from build123d import *

# Parameters (mm, degrees)
SKETCH1_W           = 14
SKETCH1_H           = 14
SKETCH1_W_2         = 9
SKETCH1_H_2         = 9
BOSS_EXTRUDE1_DEPTH = 2.5
SKETCH3_R           = 2.5
BOSS_EXTRUDE2_DEPTH = 3.4
SKETCH4_R           = 0.7
CUT_EXTRUDE1_DEPTH  = 5
FILLET1_R           = 1


with BuildPart() as part:
    # Sketch1 → Boss-Extrude1 (new body, symmetric)
    with BuildSketch(Plane.XY):
        Rectangle(SKETCH1_W, SKETCH1_H)
        Rectangle(SKETCH1_W_2, SKETCH1_H_2, mode=Mode.SUBTRACT)
    extrude(amount=BOSS_EXTRUDE1_DEPTH, both=True)

    # Sketch3 → Boss-Extrude2 (add)
    with BuildSketch(Plane(origin=(7, 0, 0), x_dir=(0, 0, -1), z_dir=(1, 0, 0))):
        Circle(SKETCH3_R)
    boss_extrude2 = extrude(amount=BOSS_EXTRUDE2_DEPTH)

    # Sketch4 → Cut-Extrude1 (cut)
    with BuildSketch(Plane(origin=(10.4, 0, 0), x_dir=(0, 0, -1), z_dir=(1, 0, 0))):
        Circle(SKETCH4_R)
    cut_extrude1 = extrude(amount=-CUT_EXTRUDE1_DEPTH, mode=Mode.SUBTRACT)

    # Mirror1: Boss-Extrude2, Cut-Extrude1 across plane
    add(boss_extrude2.mirror(Plane(origin=(0, 0, 0), x_dir=(0, 0, 1), z_dir=(1, 0, 0))))
    add(cut_extrude1.mirror(Plane(origin=(0, 0, 0), x_dir=(0, 0, 1), z_dir=(1, 0, 0))), mode=Mode.SUBTRACT)

    # Fillet1
    fillet1_edges = [part.edges().sort_by_distance(p)[0] for p in [
        (-7, 7, 0),
        (7, 7, 0),
        (7, -7, 0),
        (-7, -7, 0),
    ]]
    fillet(fillet1_edges, radius=FILLET1_R)


solid = part.part
Input: part model. Units: mm. Frame: model coordinates. A direction names the side the tool comes from. Round coordinates to 2 decimals unless told otherwise and drop trailing zeros. Order: outer loops, then holes, each group sorted by start corner. A loop starts at its lowest first (then second) coordinate and runs counter-clockwise, first axis right, second up.
1. Material intervals for line 1 (Y direction, x = 8.45, z = 0); line 2 (X direction, y = -1.5, z = -1.3); line 3 (X direction, y = -2, z = -1.9), sorted ascending.
The answers:
line 1: y = -2.5 to -0.7, 0.7 to 2.5
line 2: x = -10.4 to -4.5, 4.5 to 10.4
line 3: x = -7 to -4.5, 4.5 to 7
2. Set-up query: faces 4 (the face through (-5.4, 0, 0)), 5 (the face through (7.9, 0, 0.7)), 6 (the face through (4.5, 0, 0)). Return all of +Z, -Z, +X, -X, +Y, -Y with unobstructed straight access to the full face (end or side cutting, diameter ignored); none if empty.
The answers:
face 4: -X
face 5: +X
face 6: +Z, -Z
3. Cut plane B-B, the plane z = 0. Output: boundary loops of the cut face in (x, y).
The answers:
outline: (-10.4, -2.5) - (-7, -2.5) - (-7, -6) arc R1 ccw to (-6, -7) - (6, -7) arc R1 ccw to (7, -6) - (7, -2.5) - (10.4, -2.5) - (10.4, -0.7) - (5.4, -0.7) - (5.4, 0.7) - (10.4, 0.7) - (10.4, 2.5) - (7, 2.5) - (7, 6) arc R1 ccw to (6, 7) - (-6, 7) arc R1 ccw to (-7, 6) - (-7, 2.5) - (-10.4, 2.5) - (-10.4, 0.7) - (-5.4, 0.7) - (-5.4, -0.7) - (-10.4, -0.7) - close; hole (-4.5, -4.5) - (4.5, -4.5) - (4.5, 4.5) - (-4.5, 4.5) - close
4. Cut plane D-D, the plane x = -8. Output: boundary loops of the cut face in (y, z), then the cut area to 3 significant figures.
The answers:
outline: circle Ø5 at (0, 0); hole circle Ø1.4 at (0, 0)
area: 18.1 mm2
5. Cut plane A-A, the plane x = -4.25. Output: boundary loops of the cut face in (y, z), then the cut area to 3 significant figures.
The answers:
outline: (-7, -2.5) - (-4.5, -2.5) - (-4.5, 2.5) - (-7, 2.5) - close; (4.5, -2.5) - (7, -2.5) - (7, 2.5) - (4.5, 2.5) - close
area: 25.0 mm2
6. Pin query (flat end, axial travel): P1, Ø1.5, axis at y = -3.5, z = -1, coming from the -X side; P2, Ø0.8, axis at y = 0, z = 0, coming from the -X side; P3, Ø1.5, axis at y = 3.5, z = -0.5, coming from the +X side. Return the tip coordinate at first contact, or that it passes through.
The answers:
P1: stops at x = -7
P2: stops at x = -5.4
P3: stops at x = 7
7. Mould query, pull axis Z, two halves, no side actions, for faces 1 (the face through (8.68, -2.44, 0.54)), 2 (the face through (5.4, 0, 0)), 3 (the face through (-6.715, 6.699, -0.035)). Classes: released by +Z, released by -Z, zero draft, split by the parting line, or undercut.
The answers:
face 1: split by the parting line
face 2: undercut
face 3: zero draft
